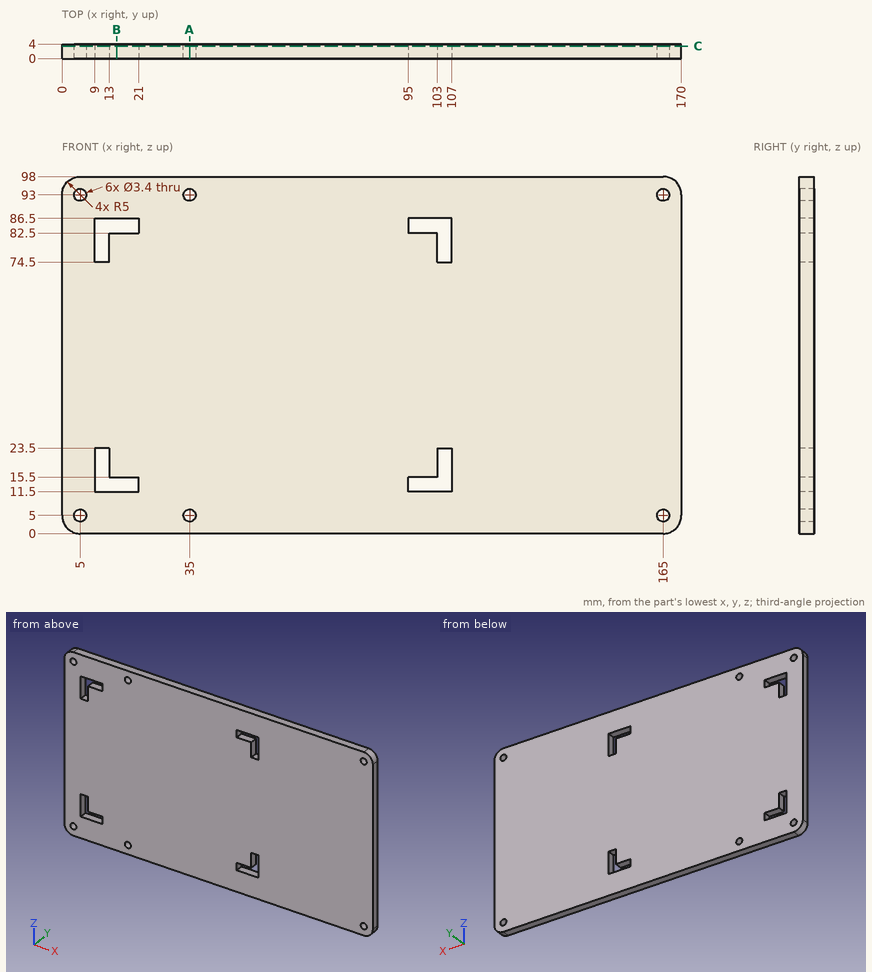
Verification items for this drawing (mm, ordinates from the low corner). Give positions to 0.01 mm unless a question says otherwise; leave off trailing zeros. Write each loop counter-clockwise with the first axis right and the second up, starting at its lowest first coordinate (ties: lowest second). Pieces come first, ordered by that corner, then holes.
1) Section check A-A, the plane x = 35. Record the boundary of the cut face in (y, z).
2) Material ranges on L1, parallel to Z at x = 5, y = 0.85; L2, parallel to X at y = 2.4, z = 80; L3, parallel to X at y = 1.75, z = 93, recorded low to high.
3) Section check C-C, the plane y = 3.4. State how many separate pieces and enclosed holes the cut face has, and give its area (3 significant figures).
4) Section check B-B, the plane x = 15. Record the boundary of the cut face in (y, z), and give its area (3 significant figures).
5) Gauge pin test, flat end, axial feed: pin 1 (3 mm diameter, centred on x = 5, z = 5, fed in from -Y). Record the tip position at first contact, or that the pin passes through.
Computed:
1. outline: (0, 0) - (4, 0) - (4, 3.3) - (0, 3.3) - close; (0, 6.7) - (4, 6.7) - (4, 91.3) - (0, 91.3) - close; (0, 94.7) - (4, 94.7) - (4, 98) - (0, 98) - close
2. L1: z = 0 to 3.3, 6.7 to 91.3, 94.7 to 98
2. L2: x = 0 to 9, 13 to 103, 107 to 170
2. L3: x = 0 to 3.3, 6.7 to 33.3, 36.7 to 163.3, 166.7 to 170
3. separate pieces: 1
3. enclosed holes: 10
3. area: 16,300 mm2
4. outline: (0, 0) - (4, 0) - (4, 11.5) - (0, 11.5) - close; (0, 15.5) - (4, 15.5) - (4, 82.5) - (0, 82.5) - close; (0, 86.5) - (4, 86.5) - (4, 98) - (0, 98) - close
4. area: 360 mm2
5. pin 1: passes through
